Work out the finished part from the listing and answer in its coordinate system (mm). Give positions to 0.01 mm unless a question says otherwise; leave off trailing zeros. Order: outer loops, then holes, each group sorted by start corner. A loop starts at its lowest first (then second) coordinate and runs counter-clockwise, first axis right, second up. Notation, with made-up numbers: (-17, 31) - (5, 31) arc R27 cw to (5, 68) - close; hole circle Ø7 at (62, 59.5). An arc over 180 degrees is marked (long way). Write each question's results on one line, items separated by ' | '.
from build123d import *

# Parameters (mm, degrees)
ESBO_O2_W                = 50
ESBO_O2_H                = 50
RESSALTO_EXTRUS_O2_DEPTH = 10
ESBO_O5_R                = 2.5
CORTE_EXTRUS_O5_DEPTH    = 37.742346142


with BuildPart() as part:
    # Esboço2 → Ressalto-extrusão2 (new body)
    with BuildSketch(Plane(origin=(0, 0, 0), x_dir=(1, 0, 0), z_dir=(0, 1, 0))):
        Rectangle(ESBO_O2_W, ESBO_O2_H)
    extrude(amount=RESSALTO_EXTRUS_O2_DEPTH)

    # Esboço5 → Corte-extrusão5 (cut, through all)
    with BuildSketch(Plane(origin=(0, 10, 0), x_dir=(1, 0, 0), z_dir=(0, 1, 0))):
        with Locations(Location((10, 18.25, 0), (0, 0, 270))):
            Circle(ESBO_O5_R)
        with Locations(Location((10, -18.25, 0), (0, 0, 270))):
            Circle(ESBO_O5_R)
    extrude(amount=-CORTE_EXTRUS_O5_DEPTH, mode=Mode.SUBTRACT)


solid = part.part
1. A cutting plane is placed at B-B, the plane z = 18.25. Write down the section's boundary in (x, y), then the cut area to 3 significant figures.
Answer list:
outline: (-25, 0) - (7.5, 0) - (7.5, 10) - (-25, 10) - close; (12.5, 0) - (25, 0) - (25, 10) - (12.5, 10) - close | area: 450 mm^2
2. A cutting plane is placed at A-A, the plane x = 10. Write down the section's boundary in (y, z), then the cut area to 3 significant figures.
Answer list:
outline: (0, -25) - (10, -25) - (10, -20.75) - (0, -20.75) - close; (0, -15.75) - (10, -15.75) - (10, 15.75) - (0, 15.75) - close; (0, 20.75) - (10, 20.75) - (10, 25) - (0, 25) - close | area: 400 mm^2
3. Determine the mould class of faces 1 (the face through (8.479, 5.07, 16.266)), 2 (the face through (25, 5, 0)), 3 (the face through (0, 5, -25)), 4 (the face through (8.479, 5.07, -20.234)) for opening direction X: +X half, -X half, draft (parallel to the pull), parting line (faces both ways), or undercut.
Answer list:
face 1: undercut | face 2: +X half | face 3: draft | face 4: undercut
4. Straight lines are drawn through the part: line 1 (X direction, y = 2, z = -18.25); line 2 (X direction, y = 2.75, z = -20). For each, find the intervals that lie inside material, in ascending order. Write a range as [from, to].
Answer list:
line 1: [-25, 7.5], [12.5, 25] | line 2: [-25, 8.21], [11.79, 25]
5. Given P1, Ø3, axis at x = 10, z = -18.25, coming from the +Y side, flat-ended and moving along its own axis, determine where the tip first touches the part or whether it passes through.
Answer list:
P1: through
6. A cutting plane is placed at C-C, the plane y = 8. Write down the section's boundary in (x, z), then the cut area to 3 significant figures.
Answer list:
outline: (-25, -25) - (25, -25) - (25, 25) - (-25, 25) - close; hole circle Ø5 at (10, -18.25); hole circle Ø5 at (10, 18.25) | area: 2,460 mm^2
